from build123d import *

# Parameters (mm, degrees)
BOSS_EXTRUDE1_DEPTH = 1.524


with BuildPart() as part:
    # Sketch1 → Boss-Extrude1 (new body)
    with BuildSketch(Plane.XY):
        with BuildLine():
            Line((4.256917141, 5.769411883), (1.572809007, 17.263448795))
            ThreePointArc((1.572809007, 17.263448795), (1.33277356, 17.653503195), (0.906545614, 17.821101488))
            ThreePointArc((0.906545614, 17.821101488), (-1.551180683, 17.70350979), (-3.936309018, 17.099018945))
            ThreePointArc((-3.936309018, 17.099018945), (-7.921935156, 15.173641861), (-11.370512849, 12.398825736))
            ThreePointArc((-11.370512849, 12.398825736), (-10.65795085, 12.520948262), (-9.945388851, 12.398825736))
            ThreePointArc((-9.945388851, 12.398825736), (-10.75175796, 11.010980832), (-11.370512849, 9.529938291))
            ThreePointArc((-11.370512849, 9.529938291), (-11.970031651, 7.843351342), (-12.427355406, 6.112786892))
            ThreePointArc((-12.427355406, 6.112786892), (-13.861120773, 1.778008598), (-14.380967646, -2.758040919))
            ThreePointArc((-14.380967646, -2.758040919), (-13.666638109, -2.037962277), (-12.676602307, -1.817487676))
            ThreePointArc((-12.676602307, -1.817487676), (-11.608509665, -5.94620724), (-9.747451479, -9.783342834))
            ThreePointArc((-9.747451479, -9.783342834), (-7.642342319, -13.987011856), (-4.222302714, -17.212790355))
            ThreePointArc((-4.222302714, -17.212790355), (-4.393060991, -16.422566374), (-4.222302714, -15.632342393))
            ThreePointArc((-4.222302714, -15.632342393), (-2.181732974, -16.682038059), (0, -17.393253279))
            ThreePointArc((0, -17.393253279), (2.054844162, -18.583773873), (4.416134447, -18.836819344))
            ThreePointArc((4.416134447, -18.836819344), (3.835913361, -18.472367282), (3.582858973, -17.835621422))
            ThreePointArc((3.582858973, -17.835621422), (6.685181318, -17.225290735), (9.400931472, -15.606152513))
            ThreePointArc((9.400931472, -15.606152513), (11.681500609, -14.751428539), (13.244817958, -12.883920166))
            ThreePointArc((13.244817958, -12.883920166), (12.377103481, -13.119413472), (11.481010343, -13.045911095))
            ThreePointArc((11.481010343, -13.045911095), (12.101156665, -11.660968144), (12.48661751, -10.193293666))
            ThreePointArc((12.48661751, -10.193293666), (12.882572593, -6.614027713), (12.879735524, -3.012928279))
            ThreePointArc((12.879735524, -3.012928279), (14.048115247, -3.839488411), (14.493985036, -5.19945641))
            ThreePointArc((14.493985036, -5.19945641), (14.133433894, -1.619098645), (12.309709537, 1.482995539))
            ThreePointArc((12.309709537, 1.482995539), (11.280344817, 5.382263311), (9.775547345, 9.123849265))
            ThreePointArc((9.775547345, 9.123849265), (11.001373452, 9.138607919), (12.138839862, 8.681401588))
            ThreePointArc((12.138839862, 8.681401588), (9.414557137, 11.619631747), (6.450200817, 14.315462683))
            ThreePointArc((6.450200817, 14.315462683), (5.574364255, 14.751975507), (4.613492818, 14.937337889))
            ThreePointArc((4.613492818, 14.937337889), (4.020029106, 14.680075469), (3.869846118, 14.050926679))
            Line((3.869846118, 14.050926679), (5.723654442, 6.111784154))
            Line((5.723654442, 6.111784154), (4.256917141, 5.769411883))
        make_face()
        with BuildLine():
            ThreePointArc((-3.040310387, 13.14603457), (-5.059685303, 11.298393601), (-6.72191547, 9.123849265))
            ThreePointArc((-6.72191547, 9.123849265), (-7.142476483, 3.70580008), (-5.728856427, -1.541466531))
            ThreePointArc((-5.728856427, -1.541466531), (-7.793494607, 0.12430808), (-9.03431247, 2.469069667))
            ThreePointArc((-9.03431247, 2.469069667), (-6.389960205, -7.924495098), (2.376676031, -14.102267879))
            ThreePointArc((2.376676031, -14.102267879), (3.21284, -13.778999141), (3.16277516, -12.883920166))
            ThreePointArc((3.16277516, -12.883920166), (-2.923149595, -0.580137917), (-3.040310387, 13.14603457))
        make_face(mode=Mode.SUBTRACT)
    extrude(amount=BOSS_EXTRUDE1_DEPTH)


solid = part.part
Can you work these out from the model? Positions are in its coordinate system, mm. A direction names the side the tool comes from. Round coordinates to 2 decimals unless told otherwise and drop trailing zeros. Write each loop counter-clockwise with the first axis right and the second up, starting at its lowest first coordinate (ties: lowest second). Pieces come first, ordered by that corner, then holes. Notation, with made-up numbers: (68.25, 87) -> (87.25, 87) arc R22 ccw to (87.25, 117) -> close; hole circle Ø10 at (4.5, 67). An arc over 180 degrees is marked (long way). One line per question, with ' | ' between items. Start each with the question number.
1) I need wall thicknesses on line 1 (X direction, y = -4.5, z = 0.2); line 2 (X direction, y = 12, z = 0.15); line 3 (X direction, y = -12.5, z = 1.15). Which ranges of each line are inside material? Lowest first, please. Write a range as [from, to].
2) Suppose I cut it at B-B on x = -7.75. Write out the boundary of the cut face in (y, z).
3) Suppose I cut it at D-D on y = 12. Write out the boundary of the cut face in (x, z), then the cut area to 3 significant figures.
4) Suppose I cut it at A-A on y = -1. Write out the boundary of the cut face in (x, z).
5) On a 3-axis mill with a long thin cutter (end or side, diameter ignored), from which of +Z, -Z, +X, -X, +Y, -Y can I reach the whole of each face in a straight line? I mean faces 4 (the cylindrical face through (5.587, 14.748, 0.751)), 5 (the flat face through (4.784, 10.137, 0.751)). Say none if no direction works.
6) If we mould it in two halves opening along Y, with no side actions, what happens to faces 1 (the cylindrical face through (-13.679, -2.045, 0.751)), 2 (the cylindrical face through (-11.96, 7.87, 0.75)), 3 (the cylindrical face through (11.298, 5.329, 0.751))? For each: released by +Y, released by -Y, zero draft, split by the parting line, or undercut.
7) Suppose I cut it at C-C on y = 4. Write out the boundary of the cut face in (x, z).
Return value:
1) line 1: x = [-12.08, -8.16], [-1.71, 12.93], [14.39, 14.55] | line 2: x = [-10.2, -4.38], [-3.27, 2.8], [4.35, 9.03] | line 3: x = [-8.6, -1.47], [2.85, 11.76]
2) outline: (-13.84, 0) -> (-5.51, 0) -> (-5.51, 1.52) -> (-13.84, 1.52) -> close; (0.07, 0) -> (15.28, 0) -> (15.28, 1.52) -> (0.07, 1.52) -> close
3) outline: (-10.2, 0) -> (-4.38, 0) -> (-4.38, 1.52) -> (-10.2, 1.52) -> close; (-3.27, 0) -> (2.8, 0) -> (2.8, 1.52) -> (-3.27, 1.52) -> close; (4.35, 0) -> (9.03, 0) -> (9.03, 1.52) -> (4.35, 1.52) -> close | area: 25.3 mm2
4) outline: (-14.29, 0) -> (-9.01, 0) -> (-9.01, 1.52) -> (-14.29, 1.52) -> close; (-6.6, 0) -> (-5.97, 0) -> (-5.97, 1.52) -> (-6.6, 1.52) -> close; (-2.82, 0) -> (13.9, 0) -> (13.9, 1.52) -> (-2.82, 1.52) -> close
5) face 4: +Z, -Z, +X, +Y | face 5: +Z, -Z
6) face 1: released by -Y | face 2: released by +Y | face 3: undercut
7) outline: (-13.25, 0) -> (-7.17, 0) -> (-7.17, 1.52) -> (-13.25, 1.52) -> close; (-3.65, 0) -> (11.7, 0) -> (11.7, 1.52) -> (-3.65, 1.52) -> close
